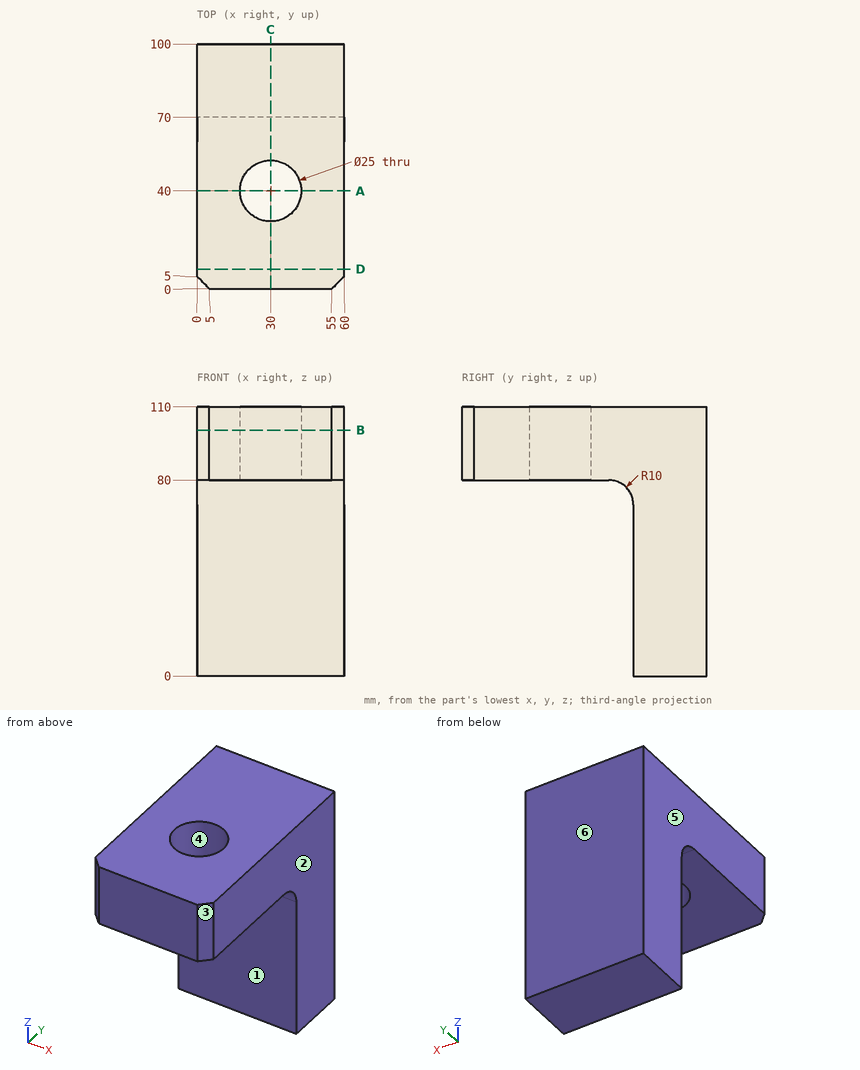
Check sheet for the drawn part. Datum: minimum x, y, z corner. Units: mm. A direction names the side the tool comes from. Round coordinates to 2 decimals unless told otherwise and drop trailing zeros. Write each loop counter-clockwise with the first axis right and the second up, starting at its lowest first coordinate (ties: lowest second). Pieces come first, ordered by that corner, then holes. Notation, with made-up numbers: (22.5, -24.5) -> (61.5, -24.5) arc R23 ccw to (61.5, -14.5) -> close; hole circle Ø10 at (87.5, -16). An arc over 180 degrees is marked (long way). Write each question's results on one line, items separated by ' | '. Start each with the question number.
1. Draft check along Y on the marked faces 3, 4, 5 and 6. Enter one of: +Y half, -Y half, draft (parallel to the pull), parting line (faces both ways), or undercut.
2. Set-up check for the marked faces 1 and 2: record each of +Z, -Z, +X, -X, +Y, -Y from which the full face is reachable in a straight line by a thin tool's end or side.
3. Cross-section at C-C (x = 30). Enter the section's corners in (y, z), then the cut area to 3 significant figures.
4. Material ranges on probe 1 along Y at (x, z) = (30, 100); probe 2 along Y at (x, z) = (8, 22); probe 3 along Y at (x, z) = (26, 84.5), recorded low to high. Write a range as from..to.
5. Cross-section at B-B (z = 100.5). Enter the section's corners in (x, y), then the cut area to 3 significant figures.
6. Cross-section at A-A (y = 40). Enter the section's corners in (x, z), then the cut area to 3 significant figures.
7. Cross-section at D-D (y = 8). Enter the section's corners in (x, z), then the cut area to 3 significant figures.
8. Depth check by flat-ended pin: P1, Ø18, axis at x = 23.5, z = 41, coming from the -Y side; P2, Ø20, axis at x = 30, y = 40, coming from the -Z side. Enter the tip coordinate at first touch or a pass-through.
Solutions:
1) face 3: -Y half | face 4: undercut | face 5: draft | face 6: +Y half
2) face 1: -Z, +X, -X, -Y | face 2: +Z, -Z, +X, +Y, -Y
3) outline: (0, 80) -> (27.5, 80) -> (27.5, 110) -> (0, 110) -> close; (52.5, 80) -> (60, 80) arc R10 cw to (70, 70) -> (70, 0) -> (100, 0) -> (100, 110) -> (52.5, 110) -> close | area: 4,670 mm2
4) probe 1: y = 0..27.5, 52.5..100 | probe 2: y = 70..100 | probe 3: y = 0..28.16, 51.84..100
5) outline: (0, 5) -> (5, 0) -> (55, 0) -> (60, 5) -> (60, 100) -> (0, 100) -> close; hole circle Ø25 at (30, 40) | area: 5,480 mm2
6) outline: (0, 80) -> (17.5, 80) -> (17.5, 110) -> (0, 110) -> close; (42.5, 80) -> (60, 80) -> (60, 110) -> (42.5, 110) -> close | area: 1,050 mm2
7) outline: (0, 80) -> (60, 80) -> (60, 110) -> (0, 110) -> close | area: 1,800 mm2
8) P1: stops at y = 70 | P2: passes through
